Verification items for the finished model (mm, model axes). Face numbers are marked on the shaded views. A direction names the side the tool comes from. Round coordinates to 2 decimals unless told otherwise and drop trailing zeros. Write each loop counter-clockwise with the first axis right and the second up, starting at its lowest first coordinate (ties: lowest second). Pieces come first, ordered by that corner, then holes. Notation, with made-up numbers: (53, 77) - (91, 77) arc R13 cw to (91, 83) - close; hole circle Ø1 at (87, -15). An arc over 180 degrees is marked (long way). Write each question's results on one line, items separated by ' | '.
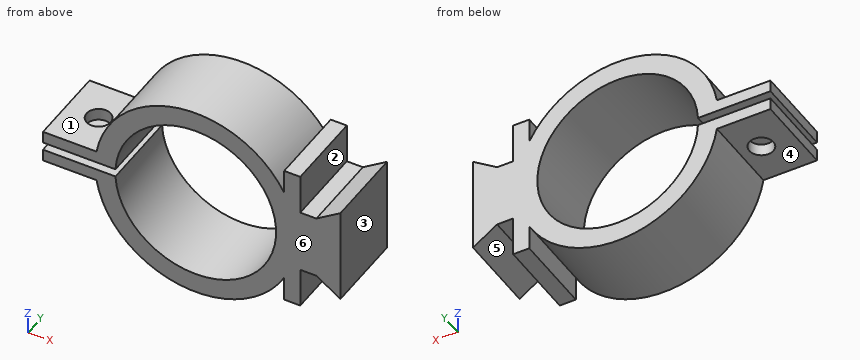
Autodesk Inventor part; units mm, degrees
ref_plane "Work Plane1" through (0, 5, 0) normal (0, 1, 0) x (1, 0, 0)
ref_plane "YZ Plane" through (0, 0, 0) normal (1, 0, 0) x (0, 1, 0)
ref_plane "XZ Plane" through (0, 0, 0) normal (0, 1, 0) x (-1, 0, 0)
sketch "Sketch1" plane through (0, 0, 0) normal (0, 1, 0) x (-1, 0, 0)
  line L0 (-0.116, 7.8509) -> (-0.116, -0.1491)
  line L1 (-0.116, -0.1491) -> (-3.116, -2.1491)
  line L2 (-3.116, -2.1491) -> (-3.116, 9.8509)
  line L3 (-0.116, 7.8509) -> (-3.116, 9.8509)
  line L4 (-0.116, 7.8509) -> (1.884, 7.8509)
  line L5 (1.884, 7.8509) -> (1.884, -0.1491)
  line L6 (1.884, -0.1491) -> (-0.116, -0.1491)
  point P0 (0, 0)
  dimension "d0" = 8
  dimension "d1" = 12
  dimension "d3" = 3
  dimension "d5" = 2
  dimension "d8" = 2
extrude "Extrusion1" add sketch "Sketch1" along normal blind 10
ref_plane "Work Plane1" through (0, 5, 0) normal (0, 1, 0) x (1, 0, 0)
sketch "Sketch2" plane through (0, 5, 0) normal (0, 1, 0) x (1, 0, 0)
  circle A0 centre (-14.884, -3.8509) radius 12.5
  line L0 (-3.884, 5.1491) -> (-1.884, 5.1491)
  line L1 (-1.884, 5.1491) -> (-1.884, -12.8509)
  line L2 (-1.884, -12.8509) -> (-3.884, -12.8509)
  line L3 (-3.884, -12.8509) -> (-3.884, 5.1491)
  line L4 (3.116, -9.8509) -> (3.116, 2.1491)
  line L5 (0.116, -7.8509) -> (3.116, -9.8509)
  line L6 (-1.884, -7.8509) -> (0.116, -7.8509)
  line L7 (-1.884, 0.1491) -> (-1.884, -7.8509)
  line L8 (0.116, 0.1491) -> (-1.884, 0.1491)
  line L9 (3.116, 2.1491) -> (0.116, 0.1491)
  line L10 (3.116, -9.8509) -> (3.116, 2.1491)
  line L11 (0.116, -7.8509) -> (3.116, -9.8509)
  line L12 (-1.884, -7.8509) -> (0.116, -7.8509)
  line L13 (-1.884, 0.1491) -> (-1.884, -7.8509)
  line L14 (0.116, 0.1491) -> (-1.884, 0.1491)
  line L15 (3.116, 2.1491) -> (0.116, 0.1491)
  circle A1 centre (-14.884, -3.8509) radius 10
  line L16 (-29.8977, -3.3509) -> (-24.5183, -3.3509)
  line L17 (-24.5183, -3.3509) -> (-24.5183, -4.3509)
  line L18 (-24.5183, -4.3509) -> (-33.884, -4.3509)
  line L19 (-33.884, -4.3509) -> (-33.884, -1.5714)
  line L20 (-29.8977, -3.3509) -> (-33.884, -3.3509)
  line L21 (-33.884, -4.3509) -> (-33.884, -5.8509)
  line L22 (-33.884, -5.8509) -> (-24.682, -5.8509)
  line L23 (-33.884, -3.3509) -> (-33.884, -1.8509)
  line L24 (-33.884, -1.8509) -> (-24.682, -1.8509)
  point P0 (0, 0)
  point P1 (-27.223, -1.8509)
  point P2 (-24.8715, -3.3509)
  point P3 (-24.8715, -4.3509)
  point P4 (-27.223, -5.8509)
  point P5 (-3.884, -9.7881)
  point P6 (-3.884, 2.0862)
  point P7 (-27.374, -4.3509)
  point P8 (-27.374, -3.3509)
  point P9 (-1.884, -7.3509)
  point P10 (-1.884, -0.3509)
  point P11 (-3.884, -3.8509)
  dimension "d9" = 25
  dimension "d10" = 0
  dimension "d11" = 5
  dimension "d12" = 5
  dimension "d13" = 2
  dimension "d14" = 9
  dimension "d15" = 20
  dimension "d16" = 13
  dimension "d17" = 1
  dimension "d18" = 1.5
  dimension "d19" = 1.5
  dimension "d26" = 0.5
  dimension "d27" = 19
extrude "Extrusion2" add sketch "Sketch2" along normal mid plane 10 contours A0 L3 | A0 L3 L0 L1 L2 | L3 A0 L22 A1 L24 | L24 A1 L16 A0 | A0 L16 L20 L19 L24 | L22 L21 L18 A0 | A0 L18 A1 L22
sketch "Sketch3" plane through (-27.223, 10, 1.8509) normal (0, 0, -1) x (-1, 0, 0)
  circle A0 centre (2.661, -4.9576) radius 1.5
  line L0 (0, 0) -> (6.661, 0)
  line L1 (0, -10) -> (0, 0)
  line L2 (6.661, -10) -> (0, -10)
  line L3 (6.661, -10) -> (6.661, 0)
  point P0 (-27.223, -10)
  dimension "d22" = 3
  dimension "d28" = 4
extrude "Extrusion3" cut sketch "Sketch3" against normal blind 10 contours A0
equation "\"d12\" = d11"
properties part number "Acople marcador_3DPrint"
(1) Section check C-C (x = -12.5). Record the cut outline in (y, z), plus the area to 3 significant figures.
Answer:
outline: (0, -8.42) - (10, -8.42) - (10, -5.86) - (0, -5.86) - close; (0, 13.56) - (10, 13.56) - (10, 16.12) - (0, 16.12) - close | area: 51.2 mm2
(2) Set-up check for the marked faces 4, 5 and 6: record each of +Z, -Z, +X, -X, +Y, -Y from which the full face is reachable in a straight line by a thin tool's end or side.
Answer:
face 4: -Z, -X, +Y, -Y | face 5: -Z, +Y, -Y | face 6: +Z, -Z, +X, -X, -Y
(3) Thickness scan on L1, parallel to X at y = 2.25, z = -3.5; L2, parallel to X at y = 6.75, z = -1.5; L3, parallel to Z at x = -28, y = 7.75. Record the ranges inside material, lowest first.
Answer:
L1: -24.99 to -21.66, -8.1 to -4.77, -3.88 to -1.88 | L2: -26.18 to -23.33, -6.44 to -1.88, 2.14 to 3.12 | L3: 1.85 to 3.35, 4.35 to 5.85
(4) Go/stop test with flat-tipped pins: pin 1 Ø1 at (x, y) = (-9.5, 5) entering from +Z; pin 2 Ø1 at (x, y) = (-3, 6.5) entering from +Z; pin 3 Ø0.9 at (y, z) = (4, -3.5) entering from -X. Record where each tip stops, or that it passes through.
Answer:
pin 1: z = 15.36 | pin 2: z = 12.85 | pin 3: x = -25.31
(5) Section check B-B (z = 11). Record the cut outline in (x, y), plus the area to 3 significant figures.
Answer:
outline: (-25.14, 0) - (-21.88, 0) - (-21.88, 10) - (-25.14, 10) - close; (-7.89, 0) - (-4.63, 0) - (-4.63, 10) - (-7.89, 10) - close; (-3.88, 0) - (-1.88, 0) - (-1.88, 10) - (-3.88, 10) - close | area: 85.2 mm2
(6) Section check D-D (y = 9.25). Record the cut outline in (x, z).
Answer:
outline: (-33.88, 1.85) - (-27.22, 1.85) arc R12.5 ccw to (-3.88, -2.09) - (-3.88, -5.15) - (-1.88, -5.15) - (-1.88, -0.15) - (0.12, -0.15) - (3.12, -2.15) - (3.12, 9.85) - (0.12, 7.85) - (-1.88, 7.85) - (-1.88, 12.85) - (-3.88, 12.85) - (-3.88, 9.79) arc R12.5 ccw to (-27.22, 5.85) - (-33.88, 5.85) - (-33.88, 4.35) - (-24.87, 4.35) arc R10 cw (long way) to (-24.87, 3.35) - (-33.88, 3.35) - close
(7) Mould release check, pull along X, two halves, no side actions. Record for the marked faces 1, 2 and 3: released by +X, released by -X, zero draft, split by the parting line, or undercut.
Answer:
face 1: zero draft | face 2: undercut | face 3: released by +X
(8) Section check A-A (y = 4). Record the cut outline in (x, z).
Answer:
outline: (-33.88, 1.85) - (-30.96, 1.85) - (-30.96, 3.35) - (-33.88, 3.35) - close; (-33.88, 4.35) - (-30.96, 4.35) - (-30.96, 5.85) - (-33.88, 5.85) - close; (-28.81, 1.85) - (-27.22, 1.85) arc R12.5 ccw to (-3.88, -2.09) - (-3.88, -5.15) - (-1.88, -5.15) - (-1.88, -0.15) - (0.12, -0.15) - (3.12, -2.15) - (3.12, 9.85) - (0.12, 7.85) - (-1.88, 7.85) - (-1.88, 12.85) - (-3.88, 12.85) - (-3.88, 9.79) arc R12.5 ccw to (-27.22, 5.85) - (-28.81, 5.85) - (-28.81, 4.35) - (-24.87, 4.35) arc R10 cw (long way) to (-24.87, 3.35) - (-28.81, 3.35) - close
